Verification items for this drawing (mm, ordinates from the low corner). A direction names the side the tool comes from. Give positions to 0.01 mm unless a question says otherwise; leave off trailing zeros. Loops run counter-clockwise (first coordinate to the right, second up) from the corner with the lowest first, then second, coordinate; pieces in that order, holes last. Notation, with made-up numbers: (65.5, 83.25) -> (73.5, 83.25) arc R8 ccw to (73.5, 88.25) -> close; hole circle Ø10 at (-9.75, 49.25). An arc over 180 degrees is marked (long way). Write each question's results on one line, items separated by ' | '. Start each with the question number.
Item 1: Cross-section at B-B on z = 6.75. Enter the section's corners in (x, y), then the cut area to 3 significant figures.
Item 2: Cross-section at D-D on x = 15.75. Enter the section's corners in (y, z).
Item 3: Access from +Z, -Z, +X, -X, +Y, -Y to the whole of each face (thin tool, end or side, straight path). Record for the marked faces 1, 2, 3 and 4.
Item 4: Cross-section at C-C on y = 69. Enter the section's corners in (x, z).
Item 5: Cross-section at A-A on x = 11. Enter the section's corners in (y, z), then the cut area to 3 significant figures.
Item 6: Gauge pin test, flat ends, axial feed: pin 1 Ø2.5 at (x, z) = (3.64, 6.75) entering from -Y; pin 2 Ø5 at (y, z) = (71, 5) entering from -X; pin 3 Ø1 at (x, z) = (6.5, 14) entering from -Y. Record the tip position at first contact, or that the pin passes through.
Item 7: Scan lines: line 1 along Z through (x, y) = (5.5, 76); line 2 along X through (y, z) = (17, 11.25). Record each from-to range of solid material in increasing order.
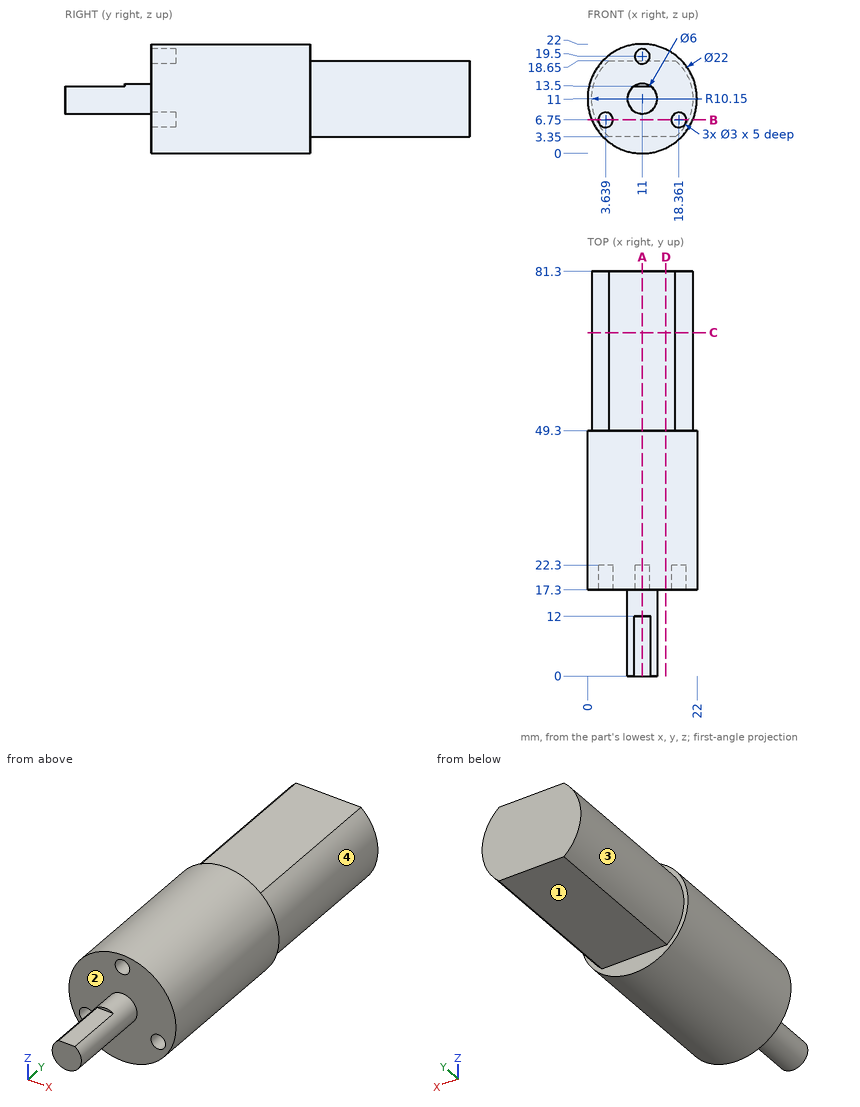
Answer sheet:
1) outline: (0.85, 17.3) -> (2.14, 17.3) -> (2.14, 22.3) -> (5.14, 22.3) -> (5.14, 17.3) -> (16.86, 17.3) -> (16.86, 22.3) -> (19.86, 22.3) -> (19.86, 17.3) -> (21.15, 17.3) -> (21.15, 49.3) -> (20.22, 49.3) -> (20.22, 81.3) -> (1.78, 81.3) -> (1.78, 49.3) -> (0.85, 49.3) -> close | area: 1,210 mm²
2) outline: (17.3, 1.08) -> (49.3, 1.08) -> (49.3, 3.35) -> (81.3, 3.35) -> (81.3, 18.65) -> (49.3, 18.65) -> (49.3, 20.92) -> (17.3, 20.92) -> close
3) face 1: -Z, +X, -X, +Y | face 2: -Y | face 3: -X, +Y | face 4: +X, +Y
4) outline: (4.33, 3.35) -> (17.67, 3.35) arc R10.15 ccw to (17.67, 18.65) -> (4.33, 18.65) arc R10.15 ccw to start
5) outline: (0, 8) -> (17.3, 8) -> (17.3, 0) -> (49.3, 0) -> (49.3, 3.35) -> (81.3, 3.35) -> (81.3, 18.65) -> (49.3, 18.65) -> (49.3, 22) -> (17.3, 22) -> (17.3, 21) -> (22.3, 21) -> (22.3, 18) -> (17.3, 18) -> (17.3, 14) -> (12, 14) -> (12, 13.5) -> (0, 13.5) -> close | area: 1,280 mm²
6) pin 1: stops at y = 22.3 | pin 2: stops at x = 1.47 | pin 3: stops at y = 17.3
7) line 1: z = 3.35 to 18.65 | line 2: x = 8.01 to 13.99
